CAD build for the part. Positions are in the model's coordinates, mm. Face numbers are marked on the shaded views. Coordinates: 2 decimals unless noted, no trailing zeros. Order: outer loops, then holes, each group sorted by start corner. A loop starts at its lowest first (then second) coordinate and runs counter-clockwise, first axis right, second up. Notation, with made-up numbers: (-19.75, -24) -> (-7.75, -24) arc R26 cw to (-7.75, 12) -> close; hole circle Ø8 at (10.5, 86). An arc over 180 degrees is marked (long way). Use one line per item in the form item = value. Start each with the question number.
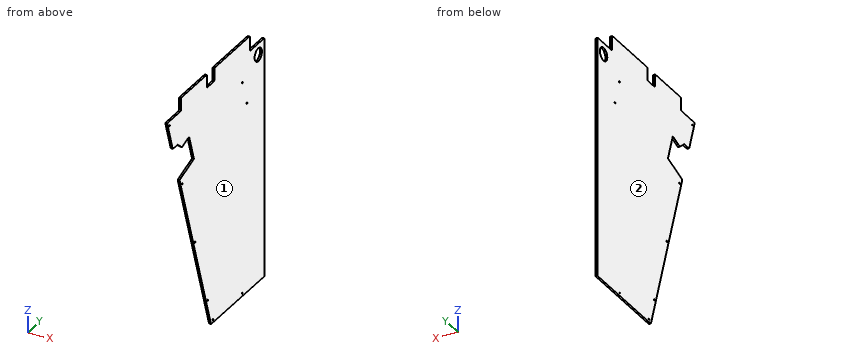
from build123d import *

# Parameters (mm, degrees)
BOSS_EXTRUDE1_DEPTH = 6.35
SKETCH2_R           = 2.45745
SKETCH2_R_2         = 22.225
SKETCH2_W           = 44.45
SKETCH2_H           = 44.45
CUT_EXTRUDE1_DEPTH  = 1236.054594947
FILLET1_R           = 3.175


with BuildPart() as part:
    # Sketch1 → Boss-Extrude1 (new body)
    with BuildSketch(Plane(origin=(0, 0, 0), x_dir=(0, 0, -1), z_dir=(1, 0, 0))):
        Polygon((1016, 533.4), (1066.8, 533.4), (1066.8, 0), (0, 0), (0, 533.4), (50.8, 533.4), (50.8, 622.3), (1016, 622.3), align=None)
    extrude(amount=BOSS_EXTRUDE1_DEPTH)

    # Sketch2 → Cut-Extrude1 (cut, through all)
    with BuildSketch(Plane(origin=(6.35, 0, 0), x_dir=(0, 0, -1), z_dir=(1, 0, 0))):
        with Locations((59.31154, 45.87748)):
            Circle(SKETCH2_R)
        with Locations((296.845703608, 123.057008284)):
            Circle(SKETCH2_R)
        with Locations((534.379867216, 200.236536569)):
            Circle(SKETCH2_R)
        with Locations((771.922083103, 277.418681197)):
            Circle(SKETCH2_R)
        with Locations((854.075, 309.0545)):
            Circle(SKETCH2_R)
        with Locations((854.075, 486.8545)):
            Circle(SKETCH2_R)
        with Locations((219.486424299, 515.220524995)):
            Circle(SKETCH2_R)
        with Locations((134.9375, 487.748914195)):
            Circle(SKETCH2_R)
        with Locations((88.9, 584.2)):
            Circle(SKETCH2_R_2)
        Polygon((149.225, 95.25), (171.033618902, 121.240499926), (157.061866823, 164.241131286), (247.65, 193.675), (276.045265579, 106.283358593), (863.6, 297.191464421), (863.6, 622.3), (1016, 622.3), (1016, 533.4), (1066.8, 533.4), (1066.8, 0), (0, 0), (0, 114.3), (44.45, 114.3), (44.45, 31.033495252), (149.225, 65.076956425), align=None)
        with Locations((22.225, 295.275)):
            Rectangle(SKETCH2_W, SKETCH2_H)
    extrude(amount=-CUT_EXTRUDE1_DEPTH, mode=Mode.SUBTRACT)

    # Fillet1
    fillet1_edges = [part.edges().sort_by_distance(p)[0] for p in [
        (3.175, 533.4, 0),
        (3.175, 533.4, -50.8),
        (3.175, 622.3, -50.8),
        (3.175, 273.05, 0),
        (3.175, 317.5, 0),
        (3.175, 317.5, -44.45),
        (3.175, 273.05, -44.45),
        (3.175, 114.3, 0),
        (3.175, 114.3, -44.45),
        (3.175, 31.033495252, -44.45),
        (3.175, 65.076956425, -149.225),
        (3.175, 95.25, -149.225),
        (3.175, 121.240499926, -171.033618902),
        (3.175, 164.241131286, -157.061866823),
        (3.175, 193.675, -247.65),
        (3.175, 106.283358593, -276.045265579),
        (3.175, 297.191464421, -863.6),
        (3.175, 622.3, -863.6),
    ]]
    fillet(fillet1_edges, radius=FILLET1_R)


solid = part.part
1) Cut at C-C on x = 5. Count the separate pieces of the cut face and the enclosed holes in it, then the cut area to 3 significant figures.
2) Cut at A-A on y = 584.2. Give the cut face in (x, z) (3 decimals), then the cut area to 3 significant figures.
3) Probe L1, parallel to Z at x = 1, y = 593; L2, parallel to Y at x = 3, z = -88.9 (3 decimals); L3, parallel to Y at x = 1.25, z = -83. List the from-to ranges inside material, lowest first.
4) Cut at B-B on z = -88.9. Give the cut face in (x, y) (3 decimals), then the cut area to 3 significant figures.
5) Cut at D-D on y = 76. Give the cut face in (x, z) (3 decimals), then the cut area to 3 significant figures.
6) Two-plate mould, pull along X, no slides. Class the marked faces 1 and 2: released by +X, released by -X, zero draft, split by the parting line, or undercut.
7) Drop flat-ended pins along their axis: P1, Ø3, axis at x = 4, y = 62.5, coming from the +Z side; P2, Ø2, axis at x = 4, z = -459, coming from the -Y side; P3, Ø2, axis at x = 4, y = 276.5, coming from the +Z side. Give the stop position or say it passes through.
Values follow:
q1.separate_pieces = 1
q1.enclosed_holes = 9
q1.area = 380,000 mm^2
q2.outline = (0, -863.6) -> (6.35, -863.6) -> (6.35, -111.125) -> (0, -111.125) -> close; (0, -66.675) -> (6.35, -66.675) -> (6.35, -50.8) -> (0, -50.8) -> close
q2.area = 4,880 mm^2
q3.L1 = -863.6 to -109.31, -68.49 to -50.8
q3.L2 = 45.476 to 561.975, 606.425 to 622.3
q3.L3 = 43.56 to 562.77, 605.63 to 622.3
q4.outline = (0, 45.476) -> (6.35, 45.476) -> (6.35, 561.975) -> (0, 561.975) -> close; (0, 606.425) -> (6.35, 606.425) -> (6.35, 622.3) -> (0, 622.3) -> close
q4.area = 3,380 mm^2
q5.outline = (0, -149.225) -> (6.35, -149.225) -> (6.35, -44.45) -> (0, -44.45) -> close
q5.area = 665 mm^2
q6.face_1 = released by +X
q6.face_2 = released by -X
q7.P1 = -44.45
q7.P2 = 165.4
q7.P3 = -44.37
